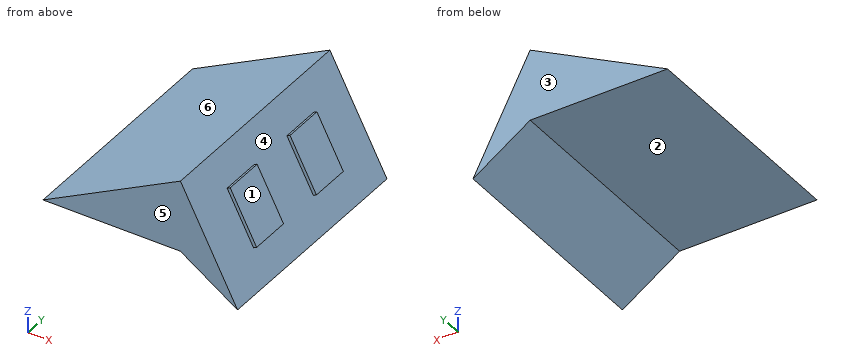
Autodesk Fusion 360 part; units mm, degrees
sketch "Esquisse1" plane through (0, 0, 0) normal (0, 1, 0) x (1, 0, 0)
  line L0 (0, 0) -> (60, 0)
  line L1 (60, 0) -> (84.9586, 16.6453)
  line L2 (84.9586, 16.6453) -> (60.0163, -31.2683)
  line L3 (60.0163, -31.2683) -> (0, 0)
  line L4 (61.2115, -4) -> (74.217, 4.6736)
  line L5 (74.217, 4.6736) -> (58.3159, -25.8721)
  line L6 (58.3159, -25.8721) -> (16.3347, -4)
  line L7 (16.3347, -4) -> (61.2115, -4)
  dimension "d1" = 60
  dimension "d2" = 30
  dimension "d3" = 146.3
  dimension "d4" = 28.8
  dimension "d5" = 54.017
  dimension "d6" = 4
extrude "Extrusion1" add sketch "Esquisse1" along normal blind 100
sketch "Esquisse2" plane through (0, 0, 0) normal (0, 1, 0) x (1, 0, 0)
  line L0 (0, 0) -> (60, 0)
  line L1 (60, 0) -> (84.9586, 16.6453)
  line L2 (84.9586, 16.6453) -> (60, -31.2598)
  line L3 (60, -31.2598) -> (0, 0)
  dimension "d9" = 60
  dimension "d10" = 146.3
  dimension "d11" = 30
  dimension "d12" = 54.017
  dimension "d13" = 28.78
sketch "Esquisse3" plane through (0, 0, 0) normal (0, 1, 0) x (1, 0, 0)
extrude "Extrusion2" add sketch "Esquisse2" along normal blind 4
sketch "Esquisse5" plane through (0, 100, 0) normal (0, 1, 0) x (-1, 0, 0)
  line L0 (-58.3159, 25.8721) -> (-16.3347, 4)
  line L1 (-16.3347, 4) -> (-61.2115, 4)
  line L2 (-61.2115, 4) -> (-74.217, -4.6736)
  line L3 (-74.217, -4.6736) -> (-58.3159, 25.8721)
  line L4 (-60.0163, 31.2683) -> (-84.9586, -16.6453)
  line L5 (-84.9586, -16.6453) -> (-60, 0)
  line L6 (-60, 0) -> (0, 0)
  line L7 (0, 0) -> (-60.0163, 31.2683)
sketch "Esquisse6" plane through (0, 100, 0) normal (0, 1, 0) x (-1, 0, 0)
  line L0 (0, 0) -> (-60, 0)
  line L1 (-60, 0) -> (-84.9586, -16.6453)
  line L2 (-84.9586, -16.6453) -> (-60.0133, 31.2668)
  line L3 (-60.0133, 31.2668) -> (0, 0)
  dimension "d21" = 60
  dimension "d22" = 146.3
  dimension "d23" = 30
  dimension "d24" = 54.017
  dimension "d25" = 28.796
extrude "Extrusion3" add sketch "Esquisse6" against normal blind 4
sketch "Esquisse7" plane through (60.0269, 0, 31.248) normal (0.887, 0, 0.4617) x (0, 1, 0)
  line L0 (0, 0.0229) -> (0, -53.9941)
  line L1 (0, -53.9941) -> (100, -53.9941)
  line L2 (100, -53.9941) -> (100, 0.0229)
  line L3 (100, 0.0229) -> (0, 0.0229)
  line L4 (39, -39.4856) -> (21, -39.4856)
  line L5 (21, -39.4856) -> (21, -14.4856)
  line L6 (21, -14.4856) -> (39, -14.4856)
  line L7 (39, -14.4856) -> (39, -39.4856)
  line L8 (39, -39.4856) -> (21, -14.4856) construction
  line L9 (21, -39.4856) -> (39, -14.4856) construction
  line L10 (61, -39.4856) -> (79, -39.4856)
  line L11 (79, -39.4856) -> (79, -14.4856)
  line L12 (79, -14.4856) -> (61, -14.4856)
  line L13 (61, -14.4856) -> (61, -39.4856)
  line L14 (61, -39.4856) -> (79, -14.4856) construction
  line L15 (79, -39.4856) -> (61, -14.4856) construction
  point P0 (30, -26.9856)
  point P1 (70, -26.9856)
  dimension "d32" = 18
  dimension "d33" = 25
  dimension "d34" = 18
  dimension "d35" = 25
extrude "Extrusion4" add sketch "Esquisse7" along normal blind 1.5 contours L4 L5 L6 L7 | L10 L11 L12 L13
Geometry check sheet. Reference: the model listing, model coordinates, mm. Face numbers are marked on the shaded views. A direction names the side the tool comes from. Round coordinates to 2 decimals unless told otherwise and drop trailing zeros. Loops run counter-clockwise (first coordinate to the right, second up) from the corner with the lowest first, then second, coordinate; pieces in that order, holes last. Notation, with made-up numbers: (83, -12.75) - (95, -12.75) arc R24 cw to (95, 20.25) - close; hole circle Ø6 at (-16.75, -15). An arc over 180 degrees is marked (long way). Write item = value, one per line. Start each with the question number.
1. Section check C-C on z = 6. Enter the section's corners in (x, y).
2. Thickness scan on line 1 (Y direction, x = 57, z = 22); line 2 (Z direction, x = 69, y = 15.5); line 3 (Z direction, x = 24, y = 28.5). Record the ranges inside material, lowest first.
3. Section check D-D on y = 29. Enter the section's corners in (x, z).
4. Set-up check for the marked faces 1 and 2: record each of +Z, -Z, +X, -X, +Y, -Y from which the full face is reachable in a straight line by a thin tool's end or side.
5. Mould release check, pull along Y, two halves, no side actions. Record for the marked faces 3, 4, 5 and 6: released by +Y, released by -Y, zero draft, split by the parting line, or undercut.
6. Section check B-B on x = 27. Enter the section's corners in (y, z).
7. Depth check by flat-ended pin: pin 1 (4 mm diameter, centred on x = 73, z = 12.5, fed in from +Y); pin 2 (1 mm diameter, centred on y = 88, z = -6, fed in from +X); pin 3 (5 mm diameter, centred on y = 65, z = 16.5, fed in from +X). Enter the tip coordinate at first touch or a pass-through.
8. Section check A-A on y = 46.5. Enter the section's corners in (x, z).
Working result:
q1.outline = (11.52, 0) - (73.17, 0) - (73.17, 21) - (74.86, 21) - (74.86, 39) - (73.17, 39) - (73.17, 61) - (74.86, 61) - (74.86, 79) - (73.17, 79) - (73.17, 100) - (11.52, 100) - close; hole (20.17, 4) - (68.66, 4) - (68.66, 96) - (20.17, 96) - close
q2.line_1 = 0 to 4, 96 to 100
q2.line_2 = -6 to -1.19, 5.35 to 14.01
q2.line_3 = 0 to 4, 7.99 to 12.5
q3.outline = (0, 0) - (60, 0) - (84.96, -16.65) - (78.26, -3.78) - (79.59, -3.08) - (68.05, 19.09) - (66.72, 18.4) - (60.02, 31.27) - close; hole (16.33, 4) - (61.21, 4) - (74.22, -4.67) - (58.32, 25.87) - close
q4.face_1 = +Z, +X, +Y, -Y
q4.face_2 = -Z, -X, +Y, -Y
q5.face_3 = released by +Y
q5.face_4 = undercut
q5.face_5 = released by -Y
q5.face_6 = zero draft
q6.outline = (0, 0) - (100, 0) - (100, 14.07) - (0, 14.07) - close; hole (4, 4) - (96, 4) - (96, 9.56) - (4, 9.56) - close
q7.pin_1 = 79
q7.pin_2 = 79.68
q7.pin_3 = 70.7
q8.outline = (0, 0) - (60, 0) - (84.96, -16.65) - (60.02, 31.27) - close; hole (16.33, 4) - (61.21, 4) - (74.22, -4.67) - (58.32, 25.87) - close
